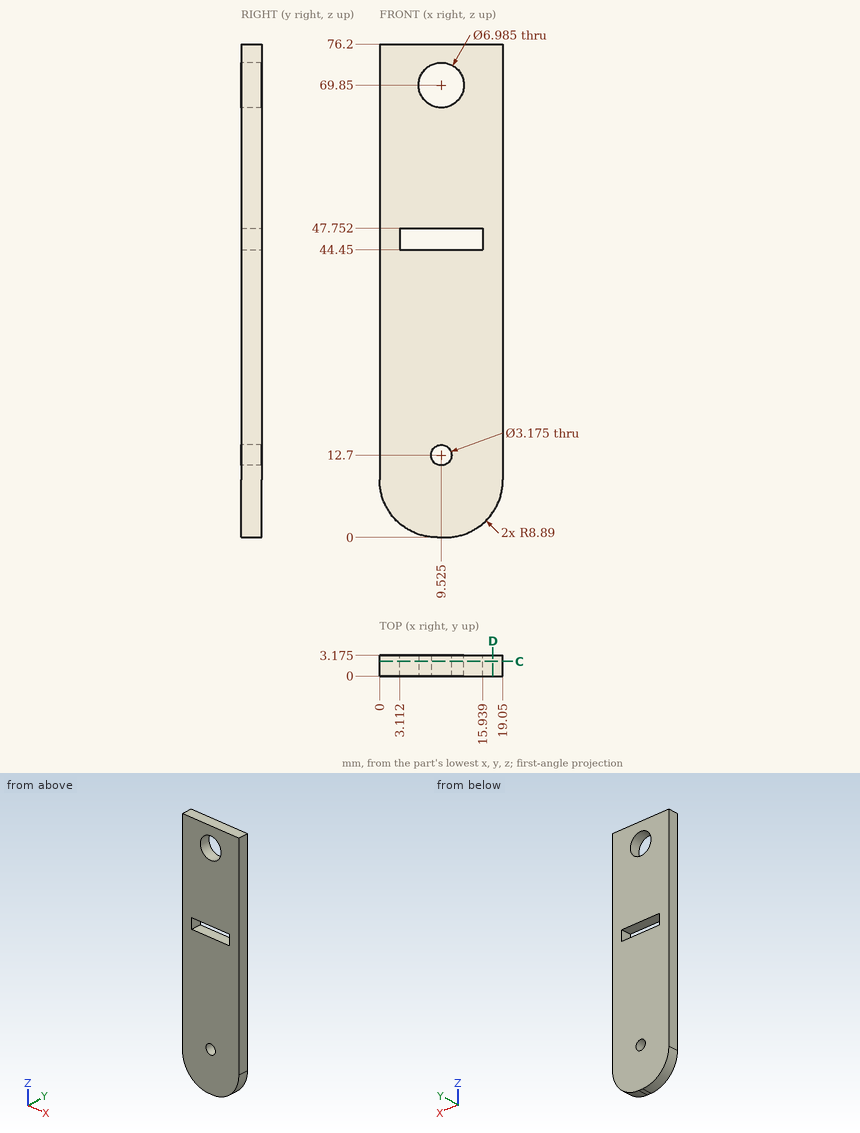
Answer from the drawing. Dimensions are ordinates in mm from the lowest x, y and z of the part. Round coordinates to 2 decimals unless told otherwise and drop trailing zeros. Write each loop counter-clockwise with the first axis right and the second up, starting at its lowest first coordinate (ties: lowest second). Pieces come first, ordered by that corner, then holes. Notation, with made-up numbers: (-28.5, 11.5) - (26.5, 11.5) arc R24 cw to (26.5, 31.5) - close; hole circle Ø3 at (75.25, 75.5). An arc over 180 degrees is marked (long way). One line per item, written item: value.
Q1. Find section D-D (x = 17.5). Determine the outline of the cut face in (y, z) (1 decimal).
The answers:
outline: (0, 3.9) - (3.2, 3.9) - (3.2, 76.2) - (0, 76.2) - close
Q2. Find section C-C (y = 2.25). Count the separate pieces of the cut face and the enclosed holes in it, and give its area (3 significant figures).
The answers:
separate pieces: 1
enclosed holes: 3
area: 1,330 mm2
Q3. This flat-tipped pin is pushed along its axis until it touches: P1, Ø3.5, axis at x = 9.525, z = 12.7, coming from the -Y side. Where does it stop, or does it pass through?
The answers:
P1: stops at y = 0
Q4. Straight lines are drawn through the part: line 1 (X direction, y = 0.85, z = 69.85); line 2 (X direction, y = 0.7, z = 45); line 3 (Z direction, x = 2.75, y = 2.4). For each, find the intervals that lie inside material, in ascending order. Write a range as from..to.
The answers:
line 1: x = 0..6.03, 13.02..19.05
line 2: x = 0..3.11, 15.94..19.05
line 3: z = 2.46..76.2
